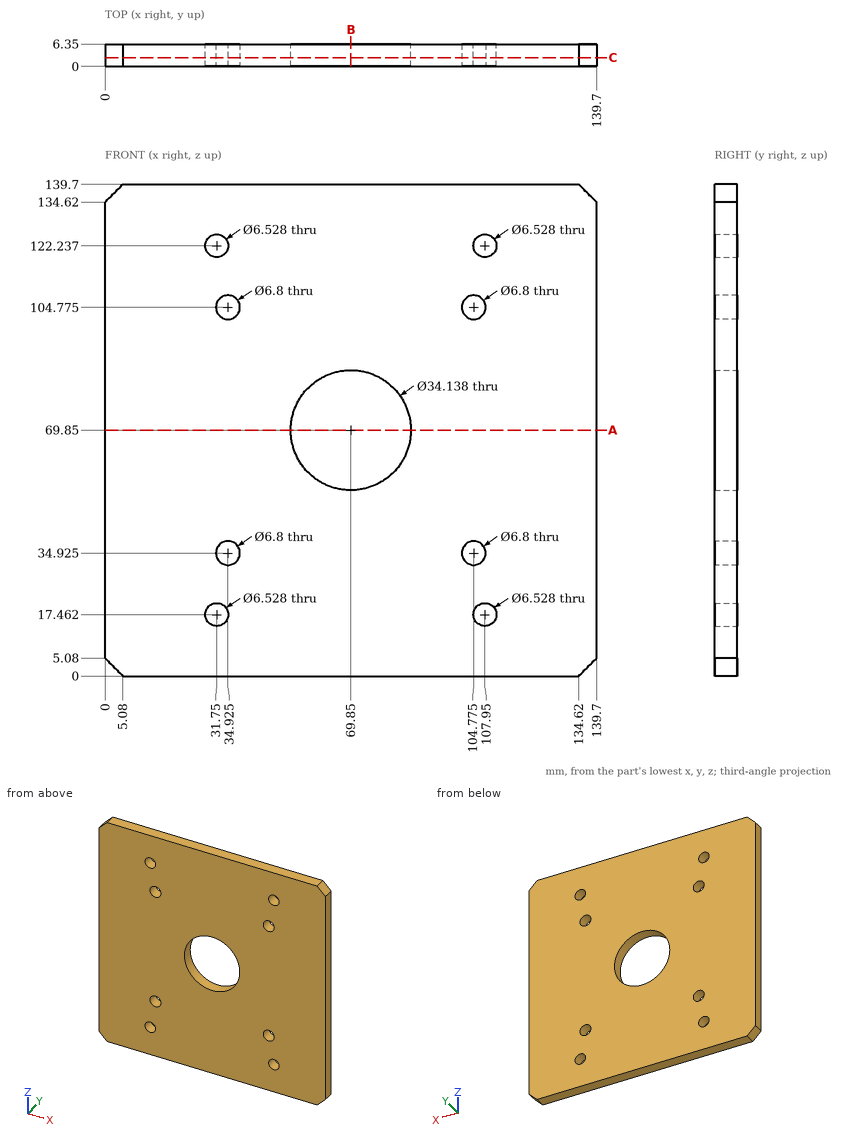
Answer from the drawing. Dimensions are ordinates in mm from the lowest x, y and z of the part. Give positions to 0.01 mm unless a question says otherwise; leave off trailing zeros. Order: outer loops, then holes, each group sorted by start corner. A loop starts at its lowest first (then second) coordinate and runs counter-clockwise, first axis right, second up. Notation, with made-up numbers: (30, 9.25) -> (87, 9.25) arc R25 cw to (87, 41.25) -> close; hole circle Ø4 at (9, 19.25). An arc over 180 degrees is marked (long way). Answer as a JSON object with one key per item and string values. Group by question number.
1. Section B-B on x = 69.85 is taken. Determine the outline of the cut face in (y, z).
2. A flat-ended cylindrical pin translates along its axis: pin 1 Ø4 at (x, z) = (107.95, 17.46) entering from -Y. Find the tip coordinate at first contact, or state that the pin passes through.
3. Section C-C on y = 2.5 is taken. Count the separate pieces of the cut face and the enclosed holes in it, plus the area to 3 significant figures.
4. Consider line 1 along Z through (x, y) = (69.85, 4.75); line 2 along X through (y, z) = (6.25, 33.5); line 3 along Z through (x, y) = (31, 6) (1 decimal). Determine where each line is inside the solid, lowest interval first. Write a range as [from, to].
5. Section A-A on z = 69.85 is taken. Determine the outline of the cut face in (x, y).
Result sheet:
{
 "1": {"outline": "(0, 0) -> (6.35, 0) -> (6.35, 52.78) -> (0, 52.78) -> close; (0, 86.92) -> (6.35, 86.92) -> (6.35, 139.7) -> (0, 139.7) -> close"},
 "2": {"pin 1": "passes through"},
 "3": {"separate pieces": "1", "enclosed holes": "9", "area": "18,300 mm^2"},
 "4": {"line 1": "z = [0, 52.78], [86.92, 139.7]", "line 2": "x = [0, 31.84], [38.01, 101.69], [107.86, 139.7]", "line 3": "z = [0, 14.3], [20.6, 119.1], [125.4, 139.7]"},
 "5": {"outline": "(0, 0) -> (52.78, 0) -> (52.78, 6.35) -> (0, 6.35) -> close; (86.92, 0) -> (139.7, 0) -> (139.7, 6.35) -> (86.92, 6.35) -> close"}
}
